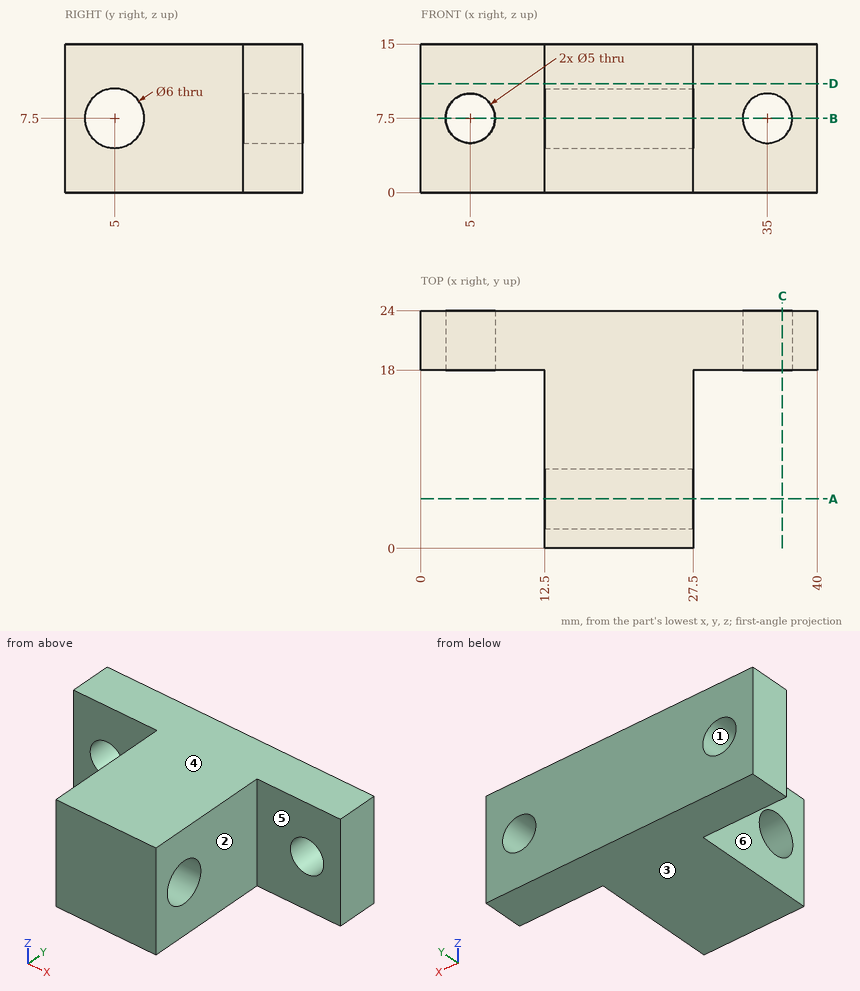
Source: three-view drawing plus pictorial views. Frame: mm from the lowest corner of the part. A direction names the side the tool comes from. Give positions to 0.01 mm unless a question says otherwise; leave off trailing zeros. Write each loop counter-clockwise with the first axis right and the second up, starting at its lowest first coordinate (ties: lowest second). Pieces come first, ordered by that corner, then holes.
(1) Cut plane B-B, the plane z = 7.5. Return loops of the section in (x, y), then the cut area to 3 significant figures.
(2) Ray query, line 1 (X direction, y = 20.8, z = 7.5); line 2 (Z direction, x = 22, y = 5); line 3 (X direction, y = 19.5, z = 8.5). Return the intervals inside material, ascending.
(3) Cut plane C-C, the plane x = 36.5. Return loops of the section in (y, z), then the cut area to 3 significant figures.
(4) Cut plane D-D, the plane z = 11. Return loops of the section in (x, y), then the cut area to 3 significant figures.
(5) First-contact query: P1, Ø7.5, axis at y = 10, z = 5, coming from the +X side; P2, Ø4.5, axis at y = 11, z = 10.5, coming from the -X side; P3, Ø6, axis at x = 36.5, z = 5.5, coming from the -Y side. Flat tips, straight axial feed; report the tip coordinate or a pass-through.
(6) Mould query, pull axis Z, two halves, no side actions, for the marked faces 1, 2 and 3. Classes: released by +Z, released by -Z, zero draft, split by the parting line, or undercut.
(7) Cut plane A-A, the plane y = 5. Return loops of the section in (x, z).
(8) Access query for the marked faces 4, 5 and 6. Directions: +Z, -Z, +X, -X, +Y, -Y. A direction counts if a zero-diameter tool reaches every point of the face in a straight line with its end or side. Return the directions, or none.
Values follow:
1. outline: (0, 18) - (2.5, 18) - (2.5, 24) - (0, 24) - close; (7.5, 18) - (12.5, 18) - (12.5, 8) - (27.5, 8) - (27.5, 18) - (32.5, 18) - (32.5, 24) - (7.5, 24) - close; (12.5, 0) - (27.5, 0) - (27.5, 2) - (12.5, 2) - close; (37.5, 18) - (40, 18) - (40, 24) - (37.5, 24) - close
1. area: 360 mm2
2. line 1: x = 0 to 2.5, 7.5 to 32.5, 37.5 to 40
2. line 2: z = 0 to 4.5, 10.5 to 15
2. line 3: x = 0 to 2.71, 7.29 to 32.71, 37.29 to 40
3. outline: (18, 0) - (24, 0) - (24, 5.5) - (18, 5.5) - close; (18, 9.5) - (24, 9.5) - (24, 15) - (18, 15) - close
3. area: 66.0 mm2
4. outline: (0, 18) - (12.5, 18) - (12.5, 0) - (27.5, 0) - (27.5, 18) - (40, 18) - (40, 24) - (0, 24) - close
4. area: 510 mm2
5. P1: stops at x = 27.5
5. P2: stops at x = 12.5
5. P3: stops at y = 18
6. face 1: undercut
6. face 2: zero draft
6. face 3: released by -Z
7. outline: (12.5, 0) - (27.5, 0) - (27.5, 4.5) - (12.5, 4.5) - close; (12.5, 10.5) - (27.5, 10.5) - (27.5, 15) - (12.5, 15) - close
8. face 4: +Z, +X, -X, +Y, -Y
8. face 5: +Z, -Z, +X, -Y
8. face 6: +Z, -Z, -X, -Y
